Could you check a few things on this model? Use its own coordinates, in mm. A direction names the side the tool comes from. Round coordinates to 2 decimals unless told otherwise and drop trailing zeros. Write each loop counter-clockwise with the first axis right and the second up, starting at its lowest first coordinate (ties: lowest second). Pieces come first, ordered by that corner, then holes. Notation, with made-up numbers: (18, 45) -> (66, 45) arc R22 cw to (66, 73) -> close; hole circle Ø6 at (-4.75, 14.25). An arc over 180 degrees is marked (long way). Return JSON: item names as keys, results as strings.
from build123d import *

# Parameters (mm, degrees)
SKETCH1_R           = 20
BOSS_EXTRUDE1_DEPTH = 32
BOSS_EXTRUDE2_DEPTH = 20
SKETCH4_R           = 8
BOSS_EXTRUDE3_DEPTH = 18
HOLE1_D             = 14
HOLE1_DEPTH         = 100


with BuildPart() as part:
    # Sketch1 → Boss-Extrude1 (new body)
    with BuildSketch(Plane.XY):
        with BuildLine():
            Line((-36, 96), (-36, 0))
            Line((-36, 0), (36, 0))
            Line((36, 0), (36, 96))
            ThreePointArc((36, 96), (0, 132), (-36, 96))
        make_face()
        with Locations((0, 96)):
            Circle(SKETCH1_R, mode=Mode.SUBTRACT)
    extrude(amount=BOSS_EXTRUDE1_DEPTH)

    # Sketch2 → Boss-Extrude2 (add)
    with BuildSketch(Plane.XY):
        with BuildLine():
            Line((36, 0), (64, 0))
            Line((64, 0), (64, 56))
            ThreePointArc((64, 56), (44.201010127, 64.201010127), (36, 84))
            Line((36, 84), (36, 0))
        make_face()
    boss_extrude2 = extrude(amount=BOSS_EXTRUDE2_DEPTH)

    # Mirror1: Boss-Extrude2 across plane
    add(boss_extrude2.mirror(Plane(origin=(0, 0, 0), x_dir=(0, 0, 1), z_dir=(1, 0, 0))))

    # Sketch4 → Boss-Extrude3 (add)
    with BuildSketch(Plane.ZY.offset(36)):
        with BuildLine():
            Line((32, 0), (92, 0))
            ThreePointArc((92, 0), (107.913745942, 14.340876714), (95.300358308, 31.65591374))
            Line((95.300358308, 31.65591374), (32, 45))
            Line((32, 45), (32, 0))
        make_face()
        with Locations(Location((92, 16, 0), (0, 0, 270))):
            Circle(SKETCH4_R, mode=Mode.SUBTRACT)
    boss_extrude3 = extrude(amount=-BOSS_EXTRUDE3_DEPTH)

    # Mirror2: Boss-Extrude3 across plane
    add(boss_extrude3.mirror(Plane(origin=(0, 0, 0), x_dir=(0, 0, 1), z_dir=(1, 0, 0))))

    # Hole1
    with Locations(Plane.XY.offset(20)):
        with Locations((54, 14), (54, 42)):
            hole1 = Hole(HOLE1_D / 2, depth=HOLE1_DEPTH)

    # Mirror3: Hole1 across plane
    add(hole1.mirror(Plane(origin=(0, 0, 0), x_dir=(0, 0, 1), z_dir=(1, 0, 0))), mode=Mode.SUBTRACT)


solid = part.part
1) I want a section at C-C, the plane x = -54. Please give me the cut outline in (y, z), and give its area (3 significant figures).
Return value:
{"outline": "(0, 0) -> (7, 0) -> (7, 20) -> (0, 20) -> close; (21, 0) -> (35, 0) -> (35, 20) -> (21, 20) -> close; (49, 0) -> (57.85, 0) -> (57.85, 20) -> (49, 20) -> close", "area": "597 mm²"}
2) I want a section at B-B, the plane y = 42. Please give me the cut outline in (x, z).
Return value:
{"outline": "(-64, 0) -> (-61, 0) -> (-61, 20) -> (-64, 20) -> close; (-47, 0) -> (47, 0) -> (47, 20) -> (36, 20) -> (36, 46.23) -> (18, 46.23) -> (18, 32) -> (-18, 32) -> (-18, 46.23) -> (-36, 46.23) -> (-36, 20) -> (-47, 20) -> close; (61, 0) -> (64, 0) -> (64, 20) -> (61, 20) -> close"}
3) For faces 1 (the face through (18, 18, 61)), 2 (the face through (-47, 33, 20)), 3 (the face through (47, 33, 20)), 4 (the face through (-1, 67, 32)), which set-ups out of +Z, -Z, +X, -X, +Y, -Y let a thin tool reach every point of the face, with its end or its side?
Return value:
{"face 1": "+Z, +Y, -Y", "face 2": "+Z, -X, +Y, -Y", "face 3": "+Z, +X, +Y, -Y", "face 4": "+Z, +Y"}
4) Will these pins go through, and if not, where does the flat tip stop? pin 1 Ø14 at (x, y) = (-55, 39.5) entering from +Z; pin 2 Ø13.5 at (y, z) = (13.5, 55.5) entering from +X; pin 3 Ø18.5 at (y, z) = (16, 92) entering from -X.
Return value:
{"pin 1": "z = 20", "pin 2": "x = 36", "pin 3": "x = -36"}
5) If I drill on probe 1 along X at (y, z) = (31, 54.5); probe 2 along Z at (x, y) = (30.5, 16); probe 3 along Y at (x, z) = (-54, 7), over which ranges is the centre line in solid material (lowest first)? Write a range as [from, to].
Return value:
{"probe 1": "[-36, -18], [18, 36]", "probe 2": "[0, 84], [100, 108]", "probe 3": "[0, 7], [21, 35], [49, 57.85]"}
6) Thinking about a two-plate mould opening in Y: for faces 5 (the face through (50.77, 7.79, 9.86)), 6 (the face through (-64, 28, 10)), 7 (the face through (-27.126, 14.014, 107.876)), which applies, pulls with the +Y half, pulls with the -Y half, needs draft (parallel to the pull), parting line crosses it, or undercut?
Return value:
{"face 5": "undercut", "face 6": "needs draft", "face 7": "parting line crosses it"}
7) I want a section at A-A, the plane x = 0. Please give me the cut outline in (y, z).
Return value:
{"outline": "(0, 0) -> (76, 0) -> (76, 32) -> (0, 32) -> close; (116, 0) -> (132, 0) -> (132, 32) -> (116, 32) -> close"}
8) I want a section at D-D, the plane y = 16. Please give me the cut outline in (x, z).
Return value:
{"outline": "(-64, 0) -> (-60.71, 0) -> (-60.71, 20) -> (-64, 20) -> close; (-47.29, 0) -> (47.29, 0) -> (47.29, 20) -> (36, 20) -> (36, 84) -> (18, 84) -> (18, 32) -> (-18, 32) -> (-18, 84) -> (-36, 84) -> (-36, 20) -> (-47.29, 20) -> close; (-36, 100) -> (-18, 100) -> (-18, 108) -> (-36, 108) -> close; (18, 100) -> (36, 100) -> (36, 108) -> (18, 108) -> close; (60.71, 0) -> (64, 0) -> (64, 20) -> (60.71, 20) -> close"}
